Verification items for this drawing (mm, ordinates from the low corner). A direction names the side the tool comes from. Give positions to 0.01 mm unless a question says otherwise; leave off trailing zeros. Loops run counter-clockwise (first coordinate to the right, second up) from the corner with the lowest first, then second, coordinate; pieces in that order, holes last. Notation, with made-up numbers: M 43.25,52.5 L 85.25,52.5 A17 ccw 85.25,65.5 Z; hole C 18,22 d3. An arc over 180 degrees is marked long. Use one line per item in the form item = value.
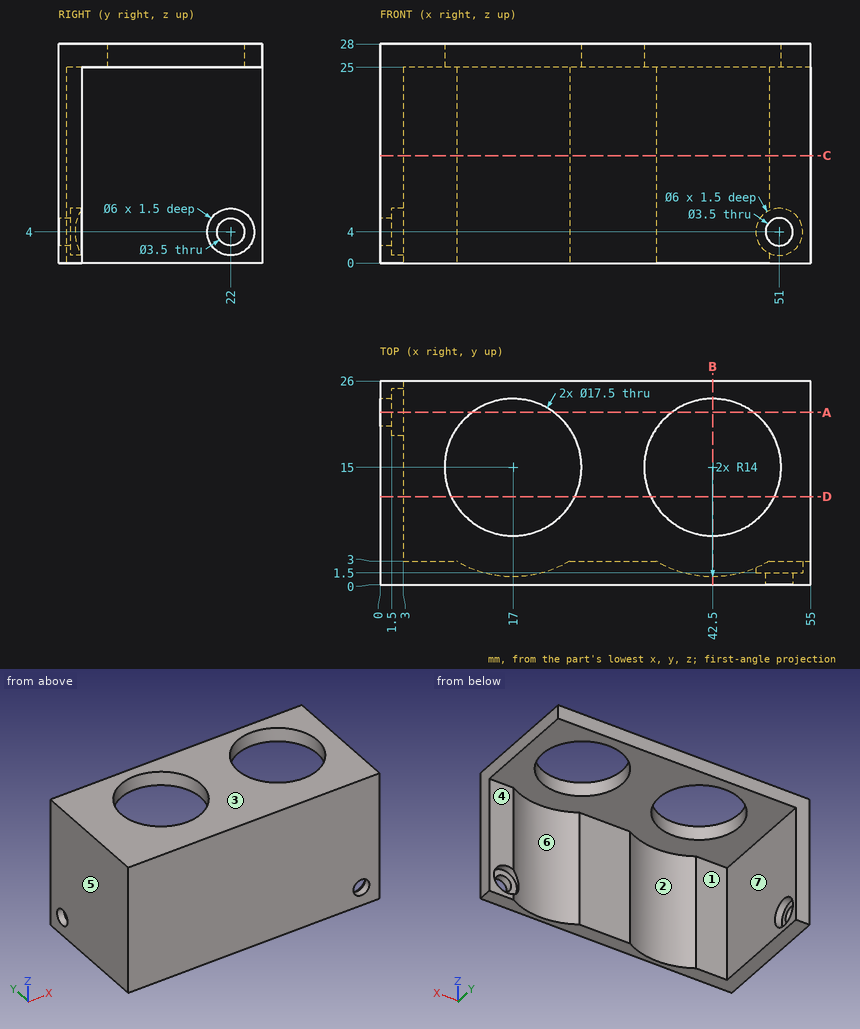
1) Section check B-B (x = 42.5). Record the cut outline in (y, z), then the cut area to 3 significant figures.
Evaluation:
outline = M 0,0 L 1,0 L 1,25 L 6.25,25 L 6.25,28 L 0,28 Z; M 23.75,25 L 26,25 L 26,28 L 23.75,28 Z
area = 50.5 mm^2
2) Section check D-D (y = 11.25). Record the cut outline in (x, z).
Evaluation:
outline = M 0,0 L 3,0 L 3,25 L 9.09,25 L 9.09,28 L 0,28 Z; M 24.91,25 L 34.59,25 L 34.59,28 L 24.91,28 Z; M 50.41,25 L 55,25 L 55,28 L 50.41,28 Z
3) Section check C-C (z = 13.75). Record the cut outline in (x, y).
Evaluation:
outline = M 0,0 L 55,0 L 55,3 L 49.71,3 A14 cw 35.29,3 L 24.21,3 A14 cw 9.79,3 L 3,3 L 3,26 L 0,26 Z
4) Scan lines: line 1 (Z direction, x = 1.1, y = 22); line 2 (Y direction, x = 2.5, z = 4); line 3 (X direction, y = 2.6, z = 4). Record each from-to range of solid material in increasing order.
Evaluation:
line_1 = 0 to 2.25, 5.75 to 28
line_2 = 0 to 19, 25 to 26
line_3 = 0 to 10.5, 23.5 to 36, 54 to 55
5) Section check A-A (y = 22). Record the cut outline in (x, z), then the cut area to 3 significant figures.
Evaluation:
outline = M 0,0 L 3,0 L 3,1 L 1.5,1 L 1.5,2.25 L 0,2.25 Z; M 0,5.75 L 1.5,5.75 L 1.5,7 L 3,7 L 3,25 L 11.75,25 L 11.75,28 L 0,28 Z; M 22.25,25 L 37.25,25 L 37.25,28 L 22.25,28 Z; M 47.75,25 L 55,25 L 55,28 L 47.75,28 Z
area = 163 mm^2
6) Set-up check for the marked faces 1, 2 and 3: record each of +Z, -Z, +X, -X, +Y, -Y from which the full face is reachable in a straight line by a thin tool's end or side.
Evaluation:
face_1 = -Z, +X, +Y
face_2 = -Z, +Y
face_3 = +Z, +X, -X, +Y, -Y
7) Depth check by flat-ended pin: pin 1 Ø4.5 at (x, z) = (51, 4) entering from -Y; pin 2 Ø7 at (x, z) = (51, 4) entering from +Y; pin 3 Ø3 at (y, z) = (23.5, 3) entering from +X; pin 4 Ø3 at (x, z) = (50.5, 3.5) entering from +Y. Enter the tip coordinate at first touch or a pass-through.
Evaluation:
pin_1 = 0
pin_2 = 3
pin_3 = 3
pin_4 = 1.5
8) Release check for a two-part mould opening along X. For the marked faces 4, 5, 6 and 7 record: pulls with the +X half, pulls with the -X half, needs draft (parallel to the pull), parting line crosses it, or undercut.
Evaluation:
face_4 = needs draft
face_5 = pulls with the -X half
face_6 = undercut
face_7 = pulls with the +X half
